```python
from build123d import *

# Parameters (mm, degrees)
F0_W     = 200
F0_H     = 57
F0_R     = 4
F1_DEPTH = 60
F2_R     = 5


with BuildPart() as f1:
    # F0 (on Top) → F1 (new body)
    with BuildSketch(Plane.XY):
        with Locations((100, 28.5)):
            Rectangle(F0_W, F0_H)
        with Locations((55, 28.5)):
            Circle(F0_R, mode=Mode.SUBTRACT)
        with Locations((112, 28.5)):
            Circle(F0_R, mode=Mode.SUBTRACT)
        with Locations((169, 28.5)):
            Circle(F0_R, mode=Mode.SUBTRACT)
    extrude(amount=F1_DEPTH)

    # F2
    f2_edges = [f1.edges().sort_by_distance(p)[0] for p in [
        (0, 0, 30),
        (100, 0, 60),
        (0, 28.5, 60),
        (100, 57, 60),
        (200, 28.5, 60),
        (200, 0, 30),
        (200, 57, 30),
        (0, 57, 30),
    ]]
    fillet(f2_edges, radius=F2_R)


solid = f1.part
```
Geometry: final body of the model. Coordinates: model frame, mm. Coordinates: 2 decimals unless noted, no trailing zeros. Order: outer loops, then holes, each group sorted by start corner. A loop starts at its lowest first (then second) coordinate and runs counter-clockwise, first axis right, second up. Notation, with made-up numbers: (79, 2) -> (112, 2) arc R26 cw to (112, 23) -> close; hole circle Ø6 at (43, 34). An arc over 180 degrees is marked (long way). Use CSV: the item, a comma, the result in double quotes.
1) Mould query, pull axis Y, two halves, no side actions, for faces 1 (the cylindrical face through (101, 56, 58)), 2 (the cylindrical face through (58.815, 29.701, 29.58)), 3 (the cylindrical face through (1, 2, 28)). Classes: +Y half, -Y half, draft (parallel to the pull), parting line (faces both ways), or undercut.
Findings:
face 1,"+Y half"
face 2,"undercut"
face 3,"-Y half"
2) Section B-B on z = 21.5. Output: boundary loops of the cut face in (x, y).
Findings:
outline,"(0, 5) arc R5 ccw to (5, 0) -> (195, 0) arc R5 ccw to (200, 5) -> (200, 52) arc R5 ccw to (195, 57) -> (5, 57) arc R5 ccw to (0, 52) -> close; hole circle Ø8 at (55, 28.5); hole circle Ø8 at (112, 28.5); hole circle Ø8 at (169, 28.5)"
3) Section D-D on x = 167.5. Output: boundary loops of the cut face in (y, z), then the cut area to 3 significant figures.
Findings:
outline,"(0, 0) -> (24.79, 0) -> (24.79, 60) -> (5, 60) arc R5 ccw to (0, 55) -> close; (32.21, 0) -> (57, 0) -> (57, 55) arc R5 ccw to (52, 60) -> (32.21, 60) -> close"
area,"2,960 mm^2"
4) Section C-C on x = 55. Output: boundary loops of the cut face in (y, z).
Findings:
outline,"(0, 0) -> (24.5, 0) -> (24.5, 60) -> (5, 60) arc R5 ccw to (0, 55) -> close; (32.5, 0) -> (57, 0) -> (57, 55) arc R5 ccw to (52, 60) -> (32.5, 60) -> close"
5) Pin query (flat end, axial travel): pin 1 Ø5 at (x, y) = (112, 28.5) entering from -Z. Return the tip coordinate at first contact, or that it passes through.
Findings:
pin 1,"passes through"
6) Line query: line 1 (Y direction, x = 112, z = 17); line 2 (Z direction, x = 128, y = 4.5); line 3 (X direction, y = 3, z = 58.5). Output: solid intervals per line, ascending.
Findings:
line 1,"y = 0 to 24.5, 32.5 to 57"
line 2,"z = 0 to 59.97"
line 3,"x = 2.04 to 197.96"
7) Section A-A on y = 28.5. Output: boundary loops of the cut face in (x, z).
Findings:
outline,"(0, 0) -> (51, 0) -> (51, 60) -> (5, 60) arc R5 ccw to (0, 55) -> close; (59, 0) -> (108, 0) -> (108, 60) -> (59, 60) -> close; (116, 0) -> (165, 0) -> (165, 60) -> (116, 60) -> close; (173, 0) -> (200, 0) -> (200, 55) arc R5 ccw to (195, 60) -> (173, 60) -> close"
